from build123d import *

# Parameters (mm, degrees)
BOSS_EXTRUDE1_DEPTH = 5
SKETCH2_R           = 2.1
CUT_EXTRUDE1_DEPTH  = 10
BOSS_EXTRUDE2_DEPTH = 5


with BuildPart() as part:
    # Sketch1 → Boss-Extrude1 (new body)
    with BuildSketch(Plane.XY):
        Polygon((-16.554054054, 7.094594595), (-21.554054054, 7.094594595), (-21.554054054, -2.905405405), (-16.554054054, -2.905405405), (-16.554054054, -0.405405405), (-11.554054054, -0.405405405), (-11.554054054, 4.594594595), (-16.554054054, 4.594594595), align=None)
    extrude(amount=BOSS_EXTRUDE1_DEPTH)

    # Sketch2 → Cut-Extrude1 (cut)
    with BuildSketch(Plane.XY.offset(5)):
        with Locations((-19.054054054, 2.094594595)):
            Circle(SKETCH2_R)
    extrude(amount=-CUT_EXTRUDE1_DEPTH, mode=Mode.SUBTRACT)

    # Sketch3 → Boss-Extrude2 (add)
    with BuildSketch(Plane.XY.offset(5)):
        with BuildLine():
            Line((-21.554054054, 5.217093594), (-21.554054054, -1.027904405))
            ThreePointArc((-21.554054054, -1.027904405), (-23.054054054, 2.094594595), (-21.554054054, 5.217093594))
        make_face()
    extrude(amount=-BOSS_EXTRUDE2_DEPTH)


solid = part.part
Geometry check sheet. Reference: the model listing, model coordinates, mm. A direction names the side the tool comes from. Give positions to 0.01 mm unless a question says otherwise; leave off trailing zeros. Write each loop counter-clockwise with the first axis right and the second up, starting at its lowest first coordinate (ties: lowest second). Pieces come first, ordered by that corner, then holes.
1) Thickness scan on line 1 (Y direction, x = -19, z = 0.65); line 2 (X direction, y = 6, z = 2.5); line 3 (X direction, y = 2, z = 2.8). Record the ranges inside material, lowest first.
Values follow:
line 1: y = -2.91 to 0, 4.19 to 7.09
line 2: x = -21.55 to -16.55
line 3: x = -23.05 to -21.15, -16.96 to -11.55
2) Cross-section at A-A (y = 0.75). Record the boundary of the cut face in (x, z), plus the area to 3 significant figures.
Values follow:
outline: (-22.82, 0) - (-20.67, 0) - (-20.67, 5) - (-22.82, 5) - close; (-17.44, 0) - (-11.55, 0) - (-11.55, 5) - (-17.44, 5) - close
area: 40.2 mm2
3) Set-up check for faces 1 (the face through (-21.554, 6, 2)), 2 (the face through (-14, 4.595, 2)), 3 (the face through (-21.554, -2, 2)), 4 (the face through (-16.554, -2, 2)): record each of +Z, -Z, +X, -X, +Y, -Y from which the full face is reachable in a straight line by a thin tool's end or side.
Values follow:
face 1: +Z, -Z, -X, +Y
face 2: +Z, -Z, +X, +Y
face 3: +Z, -Z, -X, -Y
face 4: +Z, -Z, +X, -Y
4) Cross-section at C-C (z = 1.45). Record the boundary of the cut face in (x, y), plus the area to 3 significant figures.
Values follow:
outline: (-21.55, -2.91) - (-16.55, -2.91) - (-16.55, -0.41) - (-11.55, -0.41) - (-11.55, 4.59) - (-16.55, 4.59) - (-16.55, 7.09) - (-21.55, 7.09) - (-21.55, 5.22) arc R4 ccw to (-21.55, -1.03) - close; hole circle Ø4.2 at (-19.05, 2.09)
area: 67.7 mm2
5) Cross-section at D-D (x = -12.5). Record the boundary of the cut face in (y, z), plus the area to 3 significant figures.
Values follow:
outline: (-0.41, 0) - (4.59, 0) - (4.59, 5) - (-0.41, 5) - close
area: 25.0 mm2
6) Cross-section at B-B (x = -19). Record the boundary of the cut face in (y, z), plus the area to 3 significant figures.
Values follow:
outline: (-2.91, 0) - (0, 0) - (0, 5) - (-2.91, 5) - close; (4.19, 0) - (7.09, 0) - (7.09, 5) - (4.19, 5) - close
area: 29.0 mm2
7) Go/stop test with flat-tipped pins: pin 1 Ø3.5 at (x, y) = (-19.05, 2.09) entering from -Z; pin 2 Ø2 at (x, z) = (-15, 3) entering from +Y; pin 3 Ø2.5 at (x, z) = (-15, 2) entering from -Y; pin 4 Ø1.5 at (y, z) = (6, 2.5) entering from -X. Record where each tip stops, or that it passes through.
Values follow:
pin 1: passes through
pin 2: stops at y = 4.59
pin 3: stops at y = -0.41
pin 4: stops at x = -21.55
8) Release check for a two-part mould opening along Y. For faces 5 (the face through (-16.554, 6, 2)), 6 (the face through (-19, 7.095, 2)), 7 (the face through (-21.15, 2.19, 2.54)) record: released by +Y, released by -Y, zero draft, split by the parting line, or undercut.
Values follow:
face 5: zero draft
face 6: released by +Y
face 7: undercut
